```python
from build123d import *

# Parameters (mm, degrees)
F0_W     = 15.875
F0_H     = 9.525
F1_DEPTH = 26.9875
F2_W     = 28.530914
F2_H     = 1.703672
F2_W_2   = 26.9875
F3_DEPTH = 0.508


with BuildPart() as f1:
    # F0 (on Front) → F1 (new body)
    with BuildSketch(Plane.XZ):
        Rectangle(F0_W, F0_H)
    extrude(amount=F1_DEPTH)

    # F2 (on face) → F3 (join)
    with BuildSketch(Plane.YZ.offset(7.9375)):
        with Locations((14.265457, 0.851836)):
            Rectangle(F2_W, F2_H)
        with Locations((-13.49375, 0.851836)):
            Rectangle(F2_W_2, F2_H)
        with Locations((-13.49375, -0.851836)):
            Rectangle(F2_W_2, F2_H)
        with Locations((14.265457, -0.851836)):
            Rectangle(F2_W, F2_H)
    extrude(amount=F3_DEPTH)


solid = f1.part
```
The listing builds one solid part. Answer for the finished solid, in the listing's coordinates (mm). A direction names the side the tool comes from. Coordinates: 2 decimals unless noted, no trailing zeros. Loops run counter-clockwise (first coordinate to the right, second up) from the corner with the lowest first, then second, coordinate; pieces in that order, holes last. Notation, with made-up numbers: (20.5, -35) - (67.5, -35) arc R25 cw to (67.5, -17) - close; hole circle Ø4 at (89.5, 56.25). An arc over 180 degrees is marked (long way). Use a Markdown table: item, result. Add a question column.
1) Given pin 1 (1.5 mm diameter, centred on x = -1, z = 2, fed in from +Y); pin 2 (2.5 mm diameter, centred on y = 15.5, z = 0, fed in from -X); pin 3 (0.6 mm diameter, centred on x = 8, y = 5.5, fed in from -Z), each flat-ended and moving along its own axis, determine where each tip first touches the part or whether it passes through.
2) The part is cut by section D-D, the plane y = 10. Give the vertices of the cut face in (x, z), and give its area (3 significant figures).
3) The part is cut by section C-C, the plane x = 6.25. Give the vertices of the cut face in (y, z).
4) Find the intervals of material crossed by line 1 (Y direction, x = 7, z = 0.5); line 2 (X direction, y = 24, z = -1.5); line 3 (X direction, y = -7, z = 3.25), in increasing order.
5) The part is cut by section A-A, the plane y = -18.5. Give the vertices of the cut face in (x, z), and give its area (3 significant figures).
6) For faces 1 (the flat face through (7.938, -13, 3)), 2 (the flat face through (7.938, 14, 0)), 3 (the flat face through (7.938, -13, -3)), determine the directions among +Z, -Z, +X, -X, +Y, -Y from which every point of the face is accessible in a straight line to the end or side of a thin tool.
7) The part is cut by section B-B, the plane z = 0.75. Give the vertices of the cut face in (x, y), and give its area (3 significant figures).
Here are the results:
| question | item | result |
|---|---|---|
| 1 | pin 1 | stops at y = 0 |
| 1 | pin 2 | stops at x = 7.94 |
| 1 | pin 3 | stops at z = -1.7 |
| 2 | outline | (7.94, -1.7) - (8.45, -1.7) - (8.45, 1.7) - (7.94, 1.7) - close |
| 2 | area | 1.73 mm^2 |
| 3 | outline | (-26.99, -4.76) - (0, -4.76) - (0, 4.76) - (-26.99, 4.76) - close |
| 4 | line 1 | y = -26.99 to 0 |
| 4 | line 2 | x = 7.94 to 8.45 |
| 4 | line 3 | x = -7.94 to 7.94 |
| 5 | outline | (-7.94, -4.76) - (7.94, -4.76) - (7.94, -1.7) - (8.45, -1.7) - (8.45, 1.7) - (7.94, 1.7) - (7.94, 4.76) - (-7.94, 4.76) - close |
| 5 | area | 153 mm^2 |
| 6 | face 1 | +Z, +X, +Y, -Y |
| 6 | face 2 | +Z, -Z, -X, +Y |
| 6 | face 3 | -Z, +X, +Y, -Y |
| 7 | outline | (-7.94, -26.99) - (8.45, -26.99) - (8.45, 28.53) - (7.94, 28.53) - (7.94, 0) - (-7.94, 0) - close |
| 7 | area | 457 mm^2 |
